Verification items for the finished model (mm, model axes). A direction names the side the tool comes from. Round coordinates to 2 decimals unless told otherwise and drop trailing zeros. Loops run counter-clockwise (first coordinate to the right, second up) from the corner with the lowest first, then second, coordinate; pieces in that order, holes last. Notation, with made-up numbers: (-20, 13) - (0, 13) arc R28 cw to (0, 32) - close; hole circle Ø4 at (48.5, 40). An arc over 180 degrees is marked (long way). Use CSV: the item, a comma, the result in double quotes.
```python
from build123d import *

# Parameters (mm, degrees)
F1_DEPTH = 3.175
F3_DEPTH = 1.27
F4_R     = 3.175
F5_DEPTH = 25.4


with BuildPart() as f1:
    # F0 (on Top) → F1 (new body)
    with BuildSketch(Plane.XY):
        Polygon((-76.2, 0), (0, 0), (0, 76.2), (-25.4, 76.2), (-25.4, 25.4), (-76.2, 25.4), align=None)
    extrude(amount=F1_DEPTH)

    # F2 (on face) → F3 (cut)
    with BuildSketch(Plane.XY.offset(3.175)):
        Polygon((-22.225, 76.2), (-25.4, 76.2), (-25.4, 25.4), (-76.2, 25.4), (-76.2, 22.225), (-25.4, 22.225), (-22.225, 22.225), (-22.225, 25.4), align=None)
        Polygon((-3.175, 76.2), (-19.05, 76.2), (-19.05, 19.05), (-76.2, 19.05), (-76.2, 3.175), (-19.05, 3.175), (-19.05, 0), (-3.175, 0), align=None)
    extrude(amount=-F3_DEPTH, mode=Mode.SUBTRACT)

    # F4 (on face) → F5 (cut)
    with BuildSketch(Plane.XY.offset(3.175)):
        with Locations((-12.7, 69.85)):
            Circle(F4_R)
        with Locations((-12.7, 57.15)):
            Circle(F4_R)
        with Locations((-57.15, 12.7)):
            Circle(F4_R)
        with Locations((-69.85, 12.7)):
            Circle(F4_R)
    extrude(amount=-F5_DEPTH, mode=Mode.SUBTRACT)


solid = f1.part
```
1) Cross-section at B-B, the plane y = 57.15. Record the cut outline in (x, z) (3 decimals), then the cut area to 3 significant figures.
Returned:
outline,"(-25.4, 0) - (-15.875, 0) - (-15.875, 1.905) - (-19.05, 1.905) - (-19.05, 3.175) - (-22.225, 3.175) - (-22.225, 1.905) - (-25.4, 1.905) - close; (-9.525, 0) - (0, 0) - (0, 3.175) - (-3.175, 3.175) - (-3.175, 1.905) - (-9.525, 1.905) - close"
area,"44.4 mm²"
2) Cross-section at A-A, the plane z = 2.55. Record the cut outline in (x, y) (3 decimals), then the cut area to 3 significant figures.
Returned:
outline,"(-76.2, 0) - (-19.05, 0) - (-19.05, 3.175) - (-76.2, 3.175) - close; (-76.2, 19.05) - (-19.05, 19.05) - (-19.05, 76.2) - (-22.225, 76.2) - (-22.225, 22.225) - (-76.2, 22.225) - close; (-3.175, 0) - (0, 0) - (0, 76.2) - (-3.175, 76.2) - close"
area,"776 mm²"
3) Access from +Z, -Z, +X, -X, +Y, -Y to the whole of each face (thin tool, end or side, straight path). Record for faces 5 (the face through (-25.4, 51, 1)), 6 (the face through (-13, 76.2, 1)).
Returned:
face 5,"+Z, -Z, -X, +Y"
face 6,"+Z, -Z, +X, -X, +Y"
4) Cross-section at D-D, the plane y = 34.5. Record the cut outline in (x, z) (3 decimals), then the cut area to 3 significant figures.
Returned:
outline,"(-25.4, 0) - (0, 0) - (0, 3.175) - (-3.175, 3.175) - (-3.175, 1.905) - (-19.05, 1.905) - (-19.05, 3.175) - (-22.225, 3.175) - (-22.225, 1.905) - (-25.4, 1.905) - close"
area,"56.5 mm²"
5) Mould release check, pull along X, two halves, no side actions. Record for faces 1 (the face through (-72.37, 10.77, 0.97)), 2 (the face through (-76.2, 13, 1)), 3 (the face through (0, 38, 2)), 4 (the face through (-37, 25, 1.905)): +X half, -X half, draft (parallel to the pull), parting line (faces both ways), or undercut.
Returned:
face 1,"undercut"
face 2,"-X half"
face 3,"+X half"
face 4,"draft"
6) Thickness scan on probe 1 along Y at (x, z) = (-12.7, 1.3) (3 decimals); probe 2 along X at (y, z) = (10, 1.65); probe 3 along Y at (x, z) = (-69.85, 1.05) (3 decimals). Record the ranges inside material, lowest first. Write a range as [from, to].
Returned:
probe 1,"y = [0, 53.975], [60.325, 66.675], [73.025, 76.2]"
probe 2,"x = [-76.2, -71.52], [-68.18, -58.82], [-55.48, 0]"
probe 3,"y = [0, 9.525], [15.875, 25.4]"
7) Cross-section at C-C, the plane x = -69.85. Record the cut outline in (y, z) (3 decimals), then the cut area to 3 significant figures.
Returned:
outline,"(0, 0) - (9.525, 0) - (9.525, 1.905) - (3.175, 1.905) - (3.175, 3.175) - (0, 3.175) - close; (15.875, 0) - (25.4, 0) - (25.4, 1.905) - (22.225, 1.905) - (22.225, 3.175) - (19.05, 3.175) - (19.05, 1.905) - (15.875, 1.905) - close"
area,"44.4 mm²"
8) Gauge pin test, flat ends, axial feed: pin 1 Ø1 at (x, z) = (-41.5, 0.5) entering from +Y; pin 2 Ø0.6 at (x, z) = (-42.5, 2.5) entering from +Y (3 decimals); pin 3 Ø1.5 at (y, z) = (57, 1) entering from -X; pin 4 Ø2 at (x, y) = (-46, 28) entering from -Z. Record the tip position at first contact, or that the pin passes through.
Returned:
pin 1,"stops at y = 25.4"
pin 2,"stops at y = 22.225"
pin 3,"stops at x = -25.4"
pin 4,"passes through"
